```python
from build123d import *

# Parameters (mm, degrees)
SKETCH1_W             = 26
SKETCH1_H             = 10
SKETCH1_R             = 1.5
BOSS_EXTRUDE5_DEPTH   = 3.302
SKETCH5_R             = 4.5
SKETCH5_R_2           = 3.56
BOSS_EXTRUDE7_DEPTH   = 10
SKETCH7_R             = 1.5
CUT_EXTRUDE1_DEPTH    = 10
CORTAR_EXTRUIR1_START = -10
CROQUIS1_R            = 3.56
CORTAR_EXTRUIR1_DEPTH = 10


with BuildPart() as part:
    # Sketch1 → Boss-Extrude5 (new body)
    with BuildSketch(Plane(origin=(0, 0, 0), x_dir=(1, 0, 0), z_dir=(0, 1, 0))):
        Rectangle(SKETCH1_W, SKETCH1_H)
        with Locations(Location((-9.9, 0, 0), (0, 0, 90))):
            Circle(SKETCH1_R, mode=Mode.SUBTRACT)
        with Locations(Location((9.9, 0, 0), (0, 0, 90))):
            Circle(SKETCH1_R, mode=Mode.SUBTRACT)
    extrude(amount=BOSS_EXTRUDE5_DEPTH)

    # Sketch5 → Boss-Extrude7 (add)
    with BuildSketch(Plane(origin=(0, 3.302, 0), x_dir=(1, 0, 0), z_dir=(0, 1, 0))):
        with Locations(Location((0, 0, 0), (0, 0, 90))):
            Circle(SKETCH5_R)
        with Locations(Location((0, 0, 0), (0, 0, 270))):
            Circle(SKETCH5_R_2, mode=Mode.SUBTRACT)
    extrude(amount=BOSS_EXTRUDE7_DEPTH)

    # Sketch7 → Cut-Extrude1 (cut)
    with BuildSketch(Plane(origin=(0, 0, 0), x_dir=(0, 0, -1), z_dir=(1, 0, 0))):
        with Locations(Location((0, 8.232726323, 0), (0, 0, 180))):
            Circle(SKETCH7_R)
    extrude(amount=CUT_EXTRUDE1_DEPTH, mode=Mode.SUBTRACT)

    # Croquis1 → Cortar-Extruir1 (cut)
    with BuildSketch(Plane(origin=(0, 3.302, 0), x_dir=(1, 0, 0), z_dir=(0, 1, 0)).offset(CORTAR_EXTRUIR1_START)):
        with Locations(Location((0, 0, 0), (0, 0, 90))):
            Circle(CROQUIS1_R)
    extrude(amount=CORTAR_EXTRUIR1_DEPTH, mode=Mode.SUBTRACT)


solid = part.part
```
The listing builds one solid part. Answer for the finished solid, in the listing's coordinates (mm). A direction names the side the tool comes from. Round coordinates to 2 decimals unless told otherwise and drop trailing zeros. Order: outer loops, then holes, each group sorted by start corner. A loop starts at its lowest first (then second) coordinate and runs counter-clockwise, first axis right, second up. Notation, with made-up numbers: (-10.75, -29) - (44.25, -29) arc R10 cw to (44.25, -17) - close; hole circle Ø9 at (-12, 14). An arc over 180 degrees is marked (long way). Put each result on its own line as item: value. Start each with the question number.
(1) For faces 1 (the flat face through (0, 2, 5)), 2 (the cylindrical face through (-4.46, 8.23, 0.59)), determine the directions among +Z, -Z, +X, -X, +Y, -Y from which every point of the face is accessible in a straight line to the end or side of a thin tool.
(2) Find section D-D (z = 1.75). Give the vertices of the cut face in (x, y), plus the area to 3 significant figures.
(3) Find section A-A (x = -9.9). Give the vertices of the cut face in (y, z).
(4) Determine the mould class of faces 3 (the flat face through (-3.1, 0, -2.3)), 4 (the cylindrical face through (3.856, 8.807, 1.386)), 5 (the flat face through (0, 2, -5)) for opening direction Z: released by +Z, released by -Z, zero draft, split by the parting line, or undercut.
(5) Given P1, Ø2.5, axis at x = -9.9, z = 0, coming from the -Y side; P2, Ø2, axis at x = 1.5, y = 5, coming from the +Z side; P3, Ø4, axis at y = 11, z = -1.5, coming from the +X side; P4, Ø4, axis at y = 9, z = 3.5, coming from the +X side, each flat-ended and moving along its own axis, determine where each tip first touches the part or whether it passes through.
(6) Find section B-B (z = 0). Give the vertices of the cut face in (x, y).
(7) Straight lines are drawn through the part: probe 1 along Y at (x, z) = (3.7, 0); probe 2 along Z at (x, y) = (-9.9, 0.8); probe 3 along X at (y, z) = (7.25, 2.75). For each, find the intervals that lie inside material, in ascending order. Write a range as from..to.
(8) Find section C-C (y = 1.25). Give the vertices of the cut face in (x, z).
Reply:
1. face 1: +Z, +X, -X, +Y, -Y
1. face 2: +Y
2. outline: (-13, 0) - (-3.1, 0) - (-3.1, 13.3) - (-4.15, 13.3) - (-4.15, 3.3) - (-13, 3.3) - close; (3.1, 0) - (13, 0) - (13, 3.3) - (4.15, 3.3) - (4.15, 13.3) - (3.1, 13.3) - close
2. area: 86.3 mm^2
3. outline: (0, -5) - (3.3, -5) - (3.3, -1.5) - (0, -1.5) - close; (0, 1.5) - (3.3, 1.5) - (3.3, 5) - (0, 5) - close
4. face 3: zero draft
4. face 4: undercut
4. face 5: released by -Z
5. P1: through
5. P2: z = 4.47
5. P3: x = 4.5
5. P4: x = 4.24
6. outline: (-13, 0) - (-11.4, 0) - (-11.4, 3.3) - (-13, 3.3) - close; (-8.4, 0) - (-3.56, 0) - (-3.56, 13.3) - (-4.5, 13.3) - (-4.5, 3.3) - (-8.4, 3.3) - close; (3.56, 0) - (8.4, 0) - (8.4, 3.3) - (4.5, 3.3) - (4.5, 6.73) - (3.56, 6.73) - close; (3.56, 9.73) - (4.5, 9.73) - (4.5, 13.3) - (3.56, 13.3) - close; (11.4, 0) - (13, 0) - (13, 3.3) - (11.4, 3.3) - close
7. probe 1: 0..6.73, 9.73..13.3
7. probe 2: -5..-1.5, 1.5..5
7. probe 3: -3.56..-2.26, 2.26..3.56
8. outline: (-13, -5) - (13, -5) - (13, 5) - (-13, 5) - close; hole circle Ø3 at (-9.9, 0); hole circle Ø7.12 at (0, 0); hole circle Ø3 at (9.9, 0)
